Check sheet for the modelled part. Datum: model origin and axes. Units: mm. Coordinates: 2 decimals unless noted, no trailing zeros. Loops run counter-clockwise (first coordinate to the right, second up) from the corner with the lowest first, then second, coordinate; pieces in that order, holes last. Notation, with made-up numbers: (26, 52.25) - (56, 52.25) arc R17 cw to (56, 83.25) - close; hole circle Ø2 at (-9, -11.75). An arc over 180 degrees is marked (long way). Use a Markdown table: item, result. Add a question column.
1) Sectioned sample at A-A, the plane x = 892.5. Enter the section's corners in (y, z).
2) Sectioned sample at B-B, the plane z = -100. Enter the section's corners in (x, y).
3) Thickness scan on line 1 (Y direction, x = 490, z = -305); line 2 (Y direction, x = 598, z = -476.5); line 3 (X direction, y = 50, z = -426.5). Record the ranges inside material, lowest first.
4) Go/stop test with flat-tipped pins: P1, Ø5, axis at x = 716, y = 659.5, coming from the +Z side; P2, Ø3, axis at x = 289, y = 634.5, coming from the +Z side; P3, Ø10, axis at x = 1144.5, z = -530, coming from the +Y side. Record where each tip stops, or that it passes through.
from build123d import *

# Parameters (mm, degrees)
BOSS_EXTRUDE1_DEPTH = 1016
CUT_EXTRUDE1_DEPTH  = 2287
CUT_EXTRUDE2_DEPTH  = 2287


with BuildPart() as part:
    # Sketch1 → Boss-Extrude1 (new body)
    with BuildSketch(Plane(origin=(0, 0, 0), x_dir=(1, 0, 0), z_dir=(0, 1, 0))):
        Polygon((0, 0), (0, 1016), (1778, 1016), (1778, 508), (762, 0), align=None)
    extrude(amount=BOSS_EXTRUDE1_DEPTH)

    # Sketch2 → Cut-Extrude1 (cut, through all)
    with BuildSketch(Plane(origin=(0, 0, -1016), x_dir=(-1, 0, 0), z_dir=(0, 0, -1))):
        Polygon((-762, 1016), (-1778, 508), (-1778, 1016), align=None)
    extrude(amount=-CUT_EXTRUDE1_DEPTH, mode=Mode.SUBTRACT)

    # Sketch3 → Cut-Extrude2 (cut, through all)
    with BuildSketch(Plane.ZY):
        Polygon((-508, 1016), (0, 508), (0, 1016), align=None)
    extrude(amount=-CUT_EXTRUDE2_DEPTH, mode=Mode.SUBTRACT)

    # SurfaceCut1
    split(bisect_by=Plane(origin=(197.555555556, 395.111111111, 395.111111111), x_dir=(-0.9428090415820636, 0.23570226039551598, 0.235702260395515), z_dir=(-0.33333333333333287, -0.6666666666666685, -0.6666666666666652)), keep=Keep.TOP)


solid = part.part
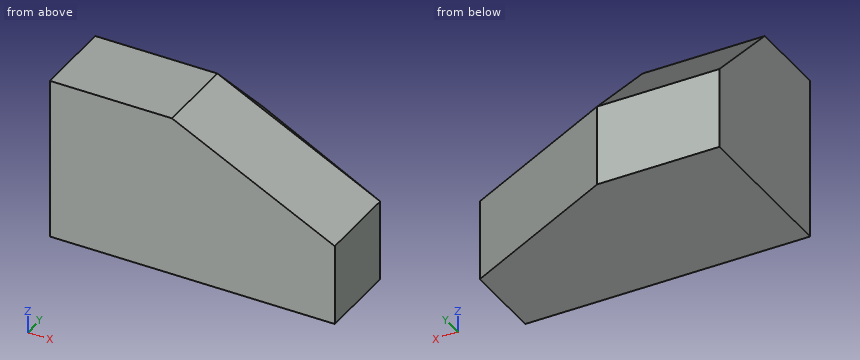
Solved:
| question | item | result |
|---|---|---|
| 1 | outline | (0, -1016) - (950.75, -1016) - (950.75, -508) - (508, -65.25) - (0, -65.25) - close |
| 2 | outline | (0, 0) - (962, 0) - (962, 508) - (762, 608) - (0, 608) - close |
| 3 | line 1 | y = 0 to 813 |
| 3 | line 2 | y = 0 to 984.5 |
| 3 | line 3 | x = 0 to 1615 |
| 4 | P1 | stops at z = -149 |
| 4 | P2 | stops at z = -125 |
| 4 | P3 | stops at y = 827.25 |
